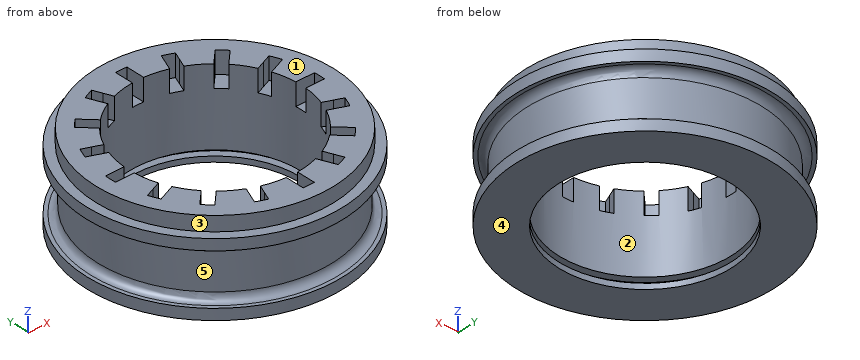
from build123d import *

# Parameters (mm, degrees)
SKETCH_1_R          = 35
SKETCH_1_R_2        = 25
SKETCH_1_R_3        = 23.5
EXTRUDE_1_DEPTH     = 10
SKETCH_3_R          = 32.5
SKETCH_3_R_2        = 23.5
EXTRUDE_2_DEPTH     = 4
CUT_EXTRUDE_1_DEPTH = 6
SKETCH_7_W          = 1.5
SKETCH_7_H          = 2


with BuildPart() as part:
    # 草图1 → 凸台-拉伸1 (new, symmetric)
    with BuildSketch(Plane.XY):
        Circle(SKETCH_1_R)
        Circle(SKETCH_1_R_2, mode=Mode.SUBTRACT)
        Circle(SKETCH_1_R_2)
        Circle(SKETCH_1_R_3, mode=Mode.SUBTRACT)
    extrude(amount=EXTRUDE_1_DEPTH, both=True)

    # 草图2 → 切除-旋转1 (revolve, cut)
    with BuildSketch(Plane(origin=(0, 0, 0), x_dir=(0, 0, -1), z_dir=(1, 0, 0)), mode=Mode.PRIVATE) as cut_revolve_1_sk:
        with BuildLine():
            Line((-7, 40), (-7, 34))
            ThreePointArc((-7, 34), (-6.414213562, 32.585786438), (-5, 32))
            Line((-5, 32), (5, 32))
            ThreePointArc((5, 32), (6.414213562, 32.585786438), (7, 34))
            Line((7, 34), (7, 40))
            Line((7, 40), (-7, 40))
        make_face()
    revolve(cut_revolve_1_sk.sketch.rotate(Axis((0, 0, 0), (0, 0, 1)), 90), axis=Axis((0, 0, 0), (0, 0, 1)), mode=Mode.SUBTRACT)

    # 草图3 → 凸台-拉伸2 (add)
    with BuildSketch(Plane.XY.offset(10)):
        Circle(SKETCH_3_R)
        Circle(SKETCH_3_R_2, mode=Mode.SUBTRACT)
    extrude(amount=EXTRUDE_2_DEPTH)

    # 草图5 → 切除-拉伸1 (cut)
    with BuildSketch(Plane.XY.offset(14)):
        with BuildLine():
            ThreePointArc((19.116635677, -21.28407168), (20.229402697, -20.229402697), (21.28407168, -19.116635677))
            Line((21.28407168, -19.116635677), (19.498162716, -17.330726713))
            Line((19.498162716, -17.330726713), (17.665351072, -15.497915069))
            ThreePointArc((17.665351072, -15.497915069), (16.623496591, -16.610519591), (15.511706041, -17.65324264))
            ThreePointArc((15.511706041, -17.65324264), (15.504811737, -17.659298202), (15.497915069, -17.665351072))
            Line((15.497915069, -17.665351072), (17.330726713, -19.498162716))
            Line((17.330726713, -19.498162716), (19.116635677, -21.28407168))
        make_face()
        with BuildLine():
            ThreePointArc((25.806530038, -12.348298438), (26.430988365, -10.948073848), (26.97953795, -9.516406827))
            Line((26.97953795, -9.516406827), (24.646135439, -8.549879861))
            Line((24.646135439, -8.549879861), (22.251451624, -7.557969347))
            ThreePointArc((22.251451624, -7.557969347), (21.71467891, -8.984582342), (21.086551211, -10.373396648))
            ThreePointArc((21.086551211, -10.373396648), (21.082499068, -10.381629594), (21.078443711, -10.389860957))
            Line((21.078443711, -10.389860957), (23.473127527, -11.381771471))
            Line((23.473127527, -11.381771471), (25.806530038, -12.348298438))
        make_face()
        with BuildLine():
            ThreePointArc((28.567614137, -1.532608696), (28.608695652, 0), (28.567614137, 1.532608696))
            Line((28.567614137, 1.532608696), (26.041957459, 1.532608696))
            Line((26.041957459, 1.532608696), (23.449970375, 1.532608696))
            ThreePointArc((23.449970375, 1.532608696), (23.487489264, 0.766712524), (23.5, 0))
            ThreePointArc((23.5, 0), (23.487786854, -0.757541226), (23.45116011, -1.514295052))
            ThreePointArc((23.45116011, -1.514295052), (23.45056703, -1.52345199), (23.449970375, -1.532608696))
            Line((23.449970375, -1.532608696), (26.041957459, -1.532608696))
            Line((26.041957459, -1.532608696), (28.567614137, -1.532608696))
        make_face()
        with BuildLine():
            ThreePointArc((26.97953795, 9.516406827), (26.430988365, 10.948073848), (25.806530038, 12.348298438))
            Line((25.806530038, 12.348298438), (23.473127527, 11.381771471))
            Line((23.473127527, 11.381771471), (21.078443711, 10.389860957))
            ThreePointArc((21.078443711, 10.389860957), (21.707655808, 9.001537608), (22.245542467, 7.575344239))
            ThreePointArc((22.245542467, 7.575344239), (22.248498741, 7.56665737), (22.251451624, 7.557969347))
            Line((22.251451624, 7.557969347), (24.646135439, 8.549879861))
            Line((24.646135439, 8.549879861), (26.97953795, 9.516406827))
        make_face()
        with BuildLine():
            ThreePointArc((21.28407168, 19.116635677), (20.229402697, 20.229402697), (19.116635677, 21.28407168))
            Line((19.116635677, 21.28407168), (17.330726713, 19.498162716))
            Line((17.330726713, 19.498162716), (15.497915069, 17.665351072))
            ThreePointArc((15.497915069, 17.665351072), (16.610519591, 16.623496591), (17.65324264, 15.511706041))
            ThreePointArc((17.65324264, 15.511706041), (17.659298202, 15.504811737), (17.665351072, 15.497915069))
            Line((17.665351072, 15.497915069), (19.498162716, 17.330726713))
            Line((19.498162716, 17.330726713), (21.28407168, 19.116635677))
        make_face()
        with BuildLine():
            Line((9.516406827, 26.97953795), (8.549879861, 24.646135439))
            Line((8.549879861, 24.646135439), (7.557969347, 22.251451624))
            ThreePointArc((7.557969347, 22.251451624), (8.984582342, 21.71467891), (10.373396648, 21.086551211))
            ThreePointArc((10.373396648, 21.086551211), (10.381629594, 21.082499068), (10.389860957, 21.078443711))
            Line((10.389860957, 21.078443711), (11.381771471, 23.473127527))
            Line((11.381771471, 23.473127527), (12.348298438, 25.806530038))
            ThreePointArc((12.348298438, 25.806530038), (10.948073848, 26.430988365), (9.516406827, 26.97953795))
        make_face()
        with BuildLine():
            ThreePointArc((1.514295052, 23.45116011), (1.52345199, 23.45056703), (1.532608696, 23.449970375))
            Line((1.532608696, 23.449970375), (1.532608696, 26.041957459))
            Line((1.532608696, 26.041957459), (1.532608696, 28.567614137))
            ThreePointArc((1.532608696, 28.567614137), (0, 28.608695652), (-1.532608696, 28.567614137))
            Line((-1.532608696, 28.567614137), (-1.532608696, 26.041957459))
            Line((-1.532608696, 26.041957459), (-1.532608696, 23.449970375))
            ThreePointArc((-1.532608696, 23.449970375), (-0.009176124, 23.499998208), (1.514295052, 23.45116011))
        make_face()
        with BuildLine():
            ThreePointArc((9.516406827, -26.97953795), (10.948073848, -26.430988365), (12.348298438, -25.806530038))
            Line((12.348298438, -25.806530038), (11.381771471, -23.473127527))
            Line((11.381771471, -23.473127527), (10.389860957, -21.078443711))
            ThreePointArc((10.389860957, -21.078443711), (9.001537608, -21.707655808), (7.575344239, -22.245542467))
            ThreePointArc((7.575344239, -22.245542467), (7.56665737, -22.248498741), (7.557969347, -22.251451624))
            Line((7.557969347, -22.251451624), (8.549879861, -24.646135439))
            Line((8.549879861, -24.646135439), (9.516406827, -26.97953795))
        make_face()
        with BuildLine():
            ThreePointArc((-1.532608696, -28.567614137), (0, -28.608695652), (1.532608696, -28.567614137))
            Line((1.532608696, -28.567614137), (1.532608696, -26.041957459))
            Line((1.532608696, -26.041957459), (1.532608696, -23.449970375))
            ThreePointArc((1.532608696, -23.449970375), (0.009176124, -23.499998208), (-1.514295052, -23.45116011))
            ThreePointArc((-1.514295052, -23.45116011), (-1.52345199, -23.45056703), (-1.532608696, -23.449970375))
            Line((-1.532608696, -23.449970375), (-1.532608696, -26.041957459))
            Line((-1.532608696, -26.041957459), (-1.532608696, -28.567614137))
        make_face()
        with BuildLine():
            Line((-11.381771471, -23.473127527), (-12.348298438, -25.806530038))
            ThreePointArc((-12.348298438, -25.806530038), (-10.948073848, -26.430988365), (-9.516406827, -26.97953795))
            Line((-9.516406827, -26.97953795), (-8.549879861, -24.646135439))
            Line((-8.549879861, -24.646135439), (-7.557969347, -22.251451624))
            ThreePointArc((-7.557969347, -22.251451624), (-8.984582342, -21.71467891), (-10.373396648, -21.086551211))
            ThreePointArc((-10.373396648, -21.086551211), (-10.381629594, -21.082499068), (-10.389860957, -21.078443711))
            Line((-10.389860957, -21.078443711), (-11.381771471, -23.473127527))
        make_face()
        with BuildLine():
            Line((-19.498162716, -17.330726713), (-21.28407168, -19.116635677))
            ThreePointArc((-21.28407168, -19.116635677), (-20.229402697, -20.229402697), (-19.116635677, -21.28407168))
            Line((-19.116635677, -21.28407168), (-17.330726713, -19.498162716))
            Line((-17.330726713, -19.498162716), (-15.497915069, -17.665351072))
            ThreePointArc((-15.497915069, -17.665351072), (-16.610519591, -16.623496591), (-17.65324264, -15.511706041))
            ThreePointArc((-17.65324264, -15.511706041), (-17.659298202, -15.504811737), (-17.665351072, -15.497915069))
            Line((-17.665351072, -15.497915069), (-19.498162716, -17.330726713))
        make_face()
        with BuildLine():
            Line((-24.646135439, -8.549879861), (-26.97953795, -9.516406827))
            ThreePointArc((-26.97953795, -9.516406827), (-26.430988365, -10.948073848), (-25.806530038, -12.348298438))
            Line((-25.806530038, -12.348298438), (-23.473127527, -11.381771471))
            Line((-23.473127527, -11.381771471), (-21.078443711, -10.389860957))
            ThreePointArc((-21.078443711, -10.389860957), (-21.707655808, -9.001537608), (-22.245542467, -7.575344239))
            ThreePointArc((-22.245542467, -7.575344239), (-22.248498741, -7.56665737), (-22.251451624, -7.557969347))
            Line((-22.251451624, -7.557969347), (-24.646135439, -8.549879861))
        make_face()
        with BuildLine():
            Line((-26.041957459, 1.532608696), (-28.567614137, 1.532608696))
            ThreePointArc((-28.567614137, 1.532608696), (-28.608695652, 0), (-28.567614137, -1.532608696))
            Line((-28.567614137, -1.532608696), (-26.041957459, -1.532608696))
            Line((-26.041957459, -1.532608696), (-23.449970375, -1.532608696))
            ThreePointArc((-23.449970375, -1.532608696), (-23.499998208, -0.009176124), (-23.45116011, 1.514295052))
            ThreePointArc((-23.45116011, 1.514295052), (-23.45056703, 1.52345199), (-23.449970375, 1.532608696))
            Line((-23.449970375, 1.532608696), (-26.041957459, 1.532608696))
        make_face()
        with BuildLine():
            Line((-23.473127527, 11.381771471), (-25.806530038, 12.348298438))
            ThreePointArc((-25.806530038, 12.348298438), (-26.430988365, 10.948073848), (-26.97953795, 9.516406827))
            Line((-26.97953795, 9.516406827), (-24.646135439, 8.549879861))
            Line((-24.646135439, 8.549879861), (-22.251451624, 7.557969347))
            ThreePointArc((-22.251451624, 7.557969347), (-21.71467891, 8.984582342), (-21.086551211, 10.373396648))
            ThreePointArc((-21.086551211, 10.373396648), (-21.082499068, 10.381629594), (-21.078443711, 10.389860957))
            Line((-21.078443711, 10.389860957), (-23.473127527, 11.381771471))
        make_face()
        with BuildLine():
            Line((-17.330726713, 19.498162716), (-19.116635677, 21.28407168))
            ThreePointArc((-19.116635677, 21.28407168), (-20.229402697, 20.229402697), (-21.28407168, 19.116635677))
            Line((-21.28407168, 19.116635677), (-19.498162716, 17.330726713))
            Line((-19.498162716, 17.330726713), (-17.665351072, 15.497915069))
            ThreePointArc((-17.665351072, 15.497915069), (-16.623496591, 16.610519591), (-15.511706041, 17.65324264))
            ThreePointArc((-15.511706041, 17.65324264), (-15.504811737, 17.659298202), (-15.497915069, 17.665351072))
            Line((-15.497915069, 17.665351072), (-17.330726713, 19.498162716))
        make_face()
        with BuildLine():
            Line((-8.549879861, 24.646135439), (-9.516406827, 26.97953795))
            ThreePointArc((-9.516406827, 26.97953795), (-10.948073848, 26.430988365), (-12.348298438, 25.806530038))
            Line((-12.348298438, 25.806530038), (-11.381771471, 23.473127527))
            Line((-11.381771471, 23.473127527), (-10.389860957, 21.078443711))
            ThreePointArc((-10.389860957, 21.078443711), (-9.001537608, 21.707655808), (-7.575344239, 22.245542467))
            ThreePointArc((-7.575344239, 22.245542467), (-7.56665737, 22.248498741), (-7.557969347, 22.251451624))
            Line((-7.557969347, 22.251451624), (-8.549879861, 24.646135439))
        make_face()
    extrude(amount=-CUT_EXTRUDE_1_DEPTH, mode=Mode.SUBTRACT)

    # 草图7 → 切除-旋转2 (revolve, cut)
    with BuildSketch(Plane(origin=(0, 0, 0), x_dir=(0, 0, -1), z_dir=(1, 0, 0)), mode=Mode.PRIVATE) as cut_revolve_2_sk:
        with Locations((7.75, 24.5)):
            Rectangle(SKETCH_7_W, SKETCH_7_H)
    revolve(cut_revolve_2_sk.sketch.rotate(Axis((0, 0, 0), (0, 0, -1)), 266.260664768), axis=Axis((0, 0, 0), (0, 0, -1)), mode=Mode.SUBTRACT)


solid = part.part
Here's how the part is built. I have some questions about the finished solid (model axes, mm). Face numbers are marked on the shaded views. A direction names the side the tool comes from. Round coordinates to 2 decimals unless told otherwise and drop trailing zeros. Loops run counter-clockwise (first coordinate to the right, second up) from the corner with the lowest first, then second, coordinate; pieces in that order, holes last.
1. If I drill on line 1 along Y through (x, z) = (0, -7.7); line 2 along Y through (x, z) = (0, 1); line 3 along Z through (x, y) = (20.5, -28), over which ranges is the centre line in solid material (lowest first)?
Answer list:
line 1: y = -35 to -25.5, 25.5 to 35
line 2: y = -32 to -23.5, 23.5 to 32
line 3: z = -10 to -7, 7 to 10
2. Which directions (+Z, -Z, +X, -X, +Y, -Y) give clear straight access to the entire face, cutting with the end or side of a thin tool? Please do the marked faces 4 and 5.
Answer list:
face 4: -Z, +X, -X, +Y, -Y
face 5: none
3. We'd pull the mould along Y, two halves only. Please class the marked faces 1, 2 and 3: +Y half, -Y half, draft (parallel to the pull), parting line (faces both ways), or undercut.
Answer list:
face 1: draft
face 2: undercut
face 3: parting line
4. For P1, Ø2.5, axis at x = -26, y = 0, coming from the +Z side; P2, Ø2.5, axis at x = 26, z = 12.5, coming from the -Y side; P3, Ø4, axis at x = -6, z = -7, coming from the -Y side, each with a flat end and sliding along its axis, tell me the tip position at first contact or that it passes through.
Answer list:
P1: stops at z = 8
P2: stops at y = -21.06
P3: stops at y = -34.77
5. If we section it at A-A on z = -3: Write out the boundary of the cut face in (x, y), plus the area to 3 significant figures.
Answer list:
outline: circle Ø64 at (0, 0); hole circle Ø47 at (0, 0)
area: 1,480 mm2
